Verification items for the finished model (mm, model axes). Coordinates: 2 decimals unless noted, no trailing zeros. Loops run counter-clockwise (first coordinate to the right, second up) from the corner with the lowest first, then second, coordinate; pieces in that order, holes last. Notation, with made-up numbers: (61.25, -40) -> (92.25, -40) arc R15 cw to (92.25, -36) -> close; hole circle Ø11 at (37, 5.25). An arc over 180 degrees is marked (long way). Answer as a JSON object with one key per item and string values. Group by question number.
Q1. Cross-section at A-A on y = 24. Record the boundary of the cut face in (x, z), and give its area (3 significant figures).
Q2. Scan lines: L1, parallel to Z at x = -4, y = -10; L2, parallel to X at y = -9.5, z = -0.5; L3, parallel to X at y = -9, z = -4.5. Record each from-to range of solid material in increasing order.
Q3. Gauge pin test, flat ends, axial feed: pin 1 Ø2 at (x, y) = (3, -5) entering from -Z; pin 2 Ø4 at (x, y) = (-1, 31.5) entering from -Z; pin 3 Ø1 at (x, y) = (-2, 21.5) entering from -Z; pin 4 Ø3 at (x, z) = (-4.5, 3) entering from -Y. Record the tip position at first contact, or that the pin passes through.
```python
from build123d import *

# Parameters (mm, degrees)
F4_DEPTH      = 1
F4_DEPTH_BACK = 1


with BuildPart() as f1:
    # F0 (on Top) → F1 (revolve)
    with BuildSketch(Plane.XY):
        with BuildLine():
            Line((0, -12.473312679), (0, 24.526687321))
            add(Edge.make_bspline(
                [(0, 24.526687321), (-1.3627446024, 23.1731329113), (-4.4742820982, 9.6920630976), (-6.3055321793, -0.6568871217), (-5.9037112934, -9.9709171664), (-2.2410321159, -12.4645982367), (0, -12.473312679)],
                knots=[0, 0, 0, 0, 0.3013061916, 0.5816044542, 0.8104723691, 1, 1, 1, 1], degree=3))
        make_face()
    revolve(axis=Axis((0, 6.026687321, 0), (0, -1, 0)))

    # F2 (on Top) → F3 (revolve)
    with BuildSketch(Plane.XY):
        with BuildLine():
            Line((0, 27.9292177189), (0, 27.4795040748))
            ThreePointArc((0, 27.4795040748), (0.5625669558, 27.5183137348), (1.1144752305, 27.6340074069))
            ThreePointArc((1.1144752305, 27.6340074069), (0.5764555854, 27.8541640655), (0, 27.9292177189))
        make_face()
        with BuildLine():
            Line((0, 27.4795040748), (0, 23.426650859))
            ThreePointArc((0, 23.426650859), (1.5918977797, 24.0860365093), (2.2512834299, 25.677934289))
            ThreePointArc((2.2512834299, 25.677934289), (1.9464424858, 26.8091454679), (1.1144752305, 27.6340074069))
            ThreePointArc((1.1144752305, 27.6340074069), (0.5625669558, 27.5183137348), (0, 27.4795040748))
        make_face()
    revolve(axis=Axis((0, 25.677934289, 0), (0, 1, 0)))

    # F2 (on Top) → F4 (join, two sides)
    with BuildSketch(Plane.XY) as f4_sk:
        with BuildLine():
            ThreePointArc((4.0967605748, 31.5762646496), (-2.4716097003, 34.8434641686), (-1.1144752305, 27.6340074069))
            ThreePointArc((-1.1144752305, 27.6340074069), (-0.5764555854, 27.8541640655), (0, 27.9292177189))
            ThreePointArc((0, 27.9292177189), (0.5764555854, 27.8541640655), (1.1144752305, 27.6340074069))
            ThreePointArc((1.1144752305, 27.6340074069), (3.2671995189, 29.1046549493), (4.0967605748, 31.5762646496))
        make_face()
        with BuildLine():
            Line((0, 27.9292177189), (0, 27.4795040748))
            ThreePointArc((0, 27.4795040748), (0.5625669558, 27.5183137348), (1.1144752305, 27.6340074069))
            ThreePointArc((1.1144752305, 27.6340074069), (0.5764555854, 27.8541640655), (0, 27.9292177189))
        make_face()
        with BuildLine():
            ThreePointArc((0, 27.9292177189), (-0.5764555854, 27.8541640655), (-1.1144752305, 27.6340074069))
            ThreePointArc((-1.1144752305, 27.6340074069), (-0.5625669558, 27.5183137348), (0, 27.4795040748))
            Line((0, 27.4795040748), (0, 27.9292177189))
        make_face()
    extrude(amount=F4_DEPTH)
    extrude(f4_sk.sketch, amount=-F4_DEPTH_BACK)


solid = f1.part
```
Computed values:
{
 "1": {"outline": "circle Ø3 at (0, 0)", "area": "7.08 mm²"},
 "2": {"L1": "z = -2.28 to 2.28", "L2": "x = -4.87 to 4.87", "L3": "x = -2.47 to 2.47"},
 "3": {"pin 1": "stops at z = -5.65", "pin 2": "stops at z = -1", "pin 3": "passes through", "pin 4": "stops at y = -10.88"}
}
